```python
from build123d import *

# Parameters (mm, degrees)
SKETCH1_R           = 85
BOSS_EXTRUDE2_DEPTH = 180
SKETCH2_W           = 90
SKETCH2_H           = 90
BOSS_EXTRUDE3_DEPTH = 50
FILLET1_R           = 20


with BuildPart() as part:
    # Sketch1 → Boss-Extrude2 (new body)
    with BuildSketch(Plane(origin=(0, 0, 0), x_dir=(1, 0, 0), z_dir=(0, 1, 0))):
        with Locations(Location((0, 0, 0), (0, 0, 90))):
            Circle(SKETCH1_R)
    extrude(amount=BOSS_EXTRUDE2_DEPTH)

    # Sketch2 → Boss-Extrude3 (add)
    with BuildSketch(Plane.XZ):
        Rectangle(SKETCH2_W, SKETCH2_H)
    extrude(amount=BOSS_EXTRUDE3_DEPTH)

    # Fillet1
    fillet1_edges = [part.edges().sort_by_distance(p)[0] for p in [
        (0, 180, 85),
    ]]
    fillet(fillet1_edges, radius=FILLET1_R)


solid = part.part
```
Can you work these out from the model? Positions are in its coordinate system, mm. A direction names the side the tool comes from. Coordinates: 2 decimals unless noted, no trailing zeros. Loops run counter-clockwise (first coordinate to the right, second up) from the corner with the lowest first, then second, coordinate; pieces in that order, holes last. Notation, with made-up numbers: (76, 10) - (100, 10) arc R17 ccw to (100, 22) - close; hole circle Ø1 at (34, 75.5). An arc over 180 degrees is marked (long way). Use a Markdown table: item, result.
Item 1: If I drill on probe 1 along Y at (x, z) = (6.5, 53.5); probe 2 along X at (y, z) = (-34, 3.5); probe 3 along X at (y, z) = (68, -22), over which ranges is the centre line in solid material (lowest first)? Write a range as from..to.
Numbers:
| item | result |
|---|---|
| probe 1 | y = 0..180 |
| probe 2 | x = -45..45 |
| probe 3 | x = -82.1..82.1 |
Item 2: For faces 1 (the face through (-1, -25, -45)), 2 (the face through (-1, -25, 45)), 3 (the face through (-45, -25, -1)), which set-ups out of +Z, -Z, +X, -X, +Y, -Y let a thin tool reach every point of the face, with its end or its side?
Numbers:
| item | result |
|---|---|
| face 1 | -Z, +X, -X, -Y |
| face 2 | +Z, +X, -X, -Y |
| face 3 | +Z, -Z, -X, -Y |
Item 3: I want a section at A-A on z = 0. Please give me the cut outline in (x, y), and give its area (3 significant figures).
Numbers:
| item | result |
|---|---|
| outline | (-85, 0) - (-45, 0) - (-45, -50) - (45, -50) - (45, 0) - (85, 0) - (85, 160) arc R20 ccw to (65, 180) - (-65, 180) arc R20 ccw to (-85, 160) - close |
| area | 34,900 mm2 |
Item 4: We'd pull the mould along Y, two halves only. Please class faces 4 (the face through (51.721, 78.88, 67.453)), 5 (the face through (-1, 180, 1)), 6 (the face through (-1, -50, 1)): released by +Y, released by -Y, zero draft, split by the parting line, or undercut.
Numbers:
| item | result |
|---|---|
| face 4 | zero draft |
| face 5 | released by +Y |
| face 6 | released by -Y |
Item 5: I want a section at C-C on y = 19. Please give me the cut outline in (x, z), and give its area (3 significant figures).
Numbers:
| item | result |
|---|---|
| outline | circle Ø170 at (0, 0) |
| area | 22,700 mm2 |
Item 6: Will these pins go through, and if not, where does the flat tip stop? pin 1 (25 mm diameter, centred on y = -17.5, z = 11.5, fed in from +X); pin 2 (1 mm diameter, centred on x = 58.5, y = 23, fed in from +Z); pin 3 (1 mm diameter, centred on x = -21.5, y = 26.5, fed in from +Z).
Numbers:
| item | result |
|---|---|
| pin 1 | stops at x = 45 |
| pin 2 | stops at z = 62.14 |
| pin 3 | stops at z = 82.37 |
Item 7: I want a section at B-B on x = 0. Please give me the cut outline in (y, z), and give its area (3 significant figures).
Numbers:
| item | result |
|---|---|
| outline | (-50, -45) - (0, -45) - (0, -85) - (160, -85) arc R20 ccw to (180, -65) - (180, 65) arc R20 ccw to (160, 85) - (0, 85) - (0, 45) - (-50, 45) - close |
| area | 34,900 mm2 |
